Part print with two shaded views. Sizes in mm from the minimum x, y, z corner. Give positions to 0.01 mm unless a question says otherwise; leave off trailing zeros. Order: outer loops, then holes, each group sorted by start corner. A loop starts at its lowest first (then second) coordinate and runs counter-clockwise, first axis right, second up.
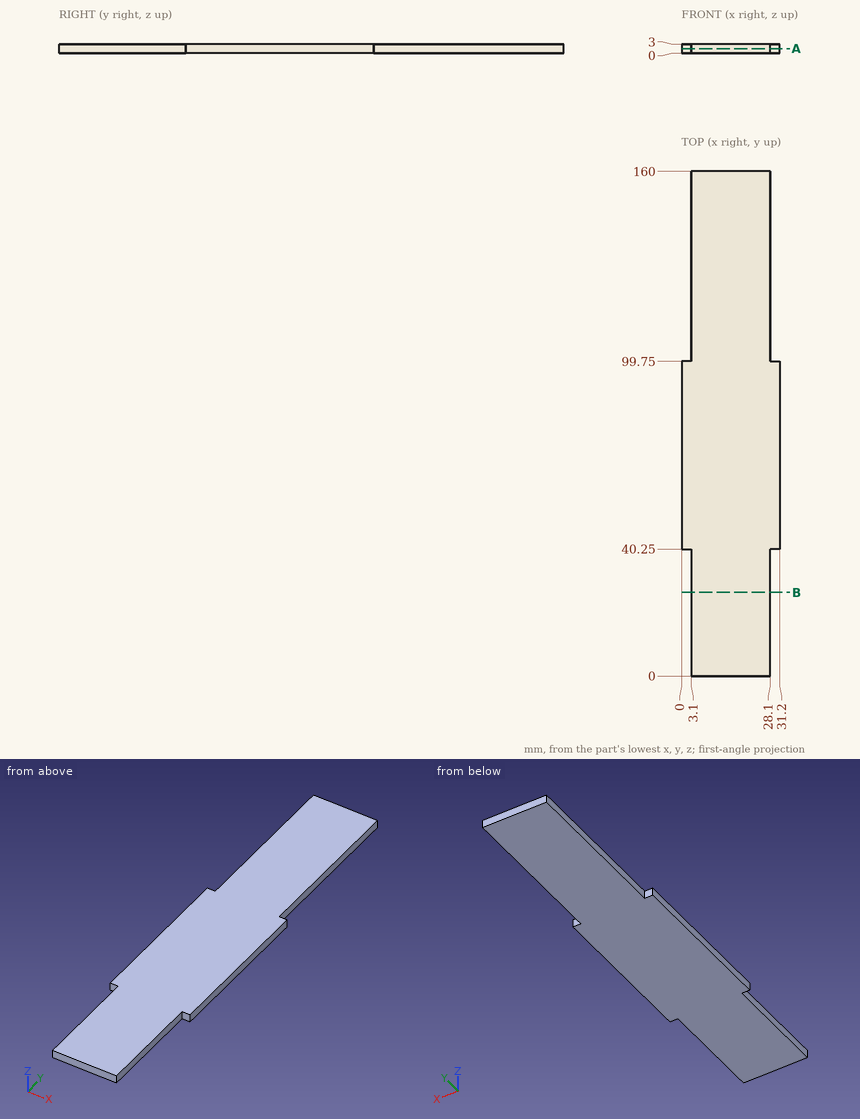
1. Wall check: line 1 (Y direction, x = 29.5, z = 0.95); line 2 (X direction, y = 39, z = 1.9). Give the ranges that are in metal, low to high.
2. Saw through at A-A on z = 1.55. Give the cut face in (x, y).
3. Pin check, flat tips, straight feed: P1, Ø0.9, axis at y = 130.5, z = 1.5, coming from the -X side; P2, Ø0.9, axis at y = 137.5, z = 1.5, coming from the +X side; P3, Ø0.9, axis at x = 2, z = 1.5, coming from the -Y side. Stop position of each tip, or through.
4. Saw through at B-B on y = 26.5. Give the cut face in (x, z), plus the area to 3 significant figures.
Reported:
1. line 1: y = 40.25 to 99.75
1. line 2: x = 3.1 to 28.1
2. outline: (0, 40.25) - (3.1, 40.25) - (3.1, 0) - (28.1, 0) - (28.1, 40.25) - (31.2, 40.25) - (31.2, 99.75) - (28.1, 99.75) - (28.1, 160) - (3.1, 160) - (3.1, 99.75) - (0, 99.75) - close
3. P1: stops at x = 3.1
3. P2: stops at x = 28.1
3. P3: stops at y = 40.25
4. outline: (3.1, 0) - (28.1, 0) - (28.1, 3) - (3.1, 3) - close
4. area: 75.0 mm2
